Read the model definition and answer for the solid it produces. Units are mm, in the model's axes. Round coordinates to 2 decimals unless told otherwise and drop trailing zeros. Write each loop counter-clockwise with the first axis right and the second up, starting at its lowest first coordinate (ties: lowest second). Pieces come first, ordered by that corner, then holes.
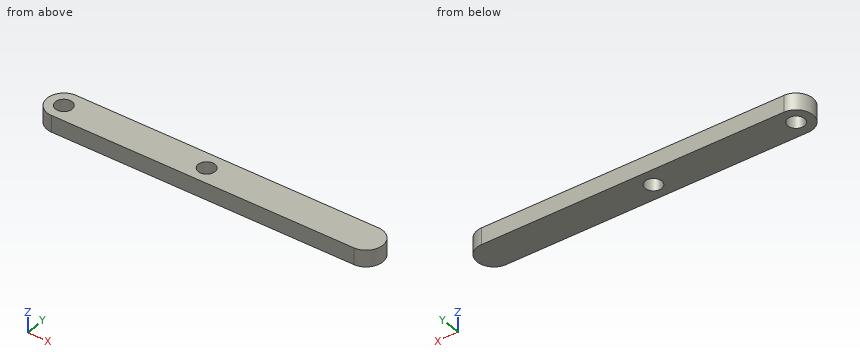
Autodesk Inventor part; units mm, degrees
ref_plane "YZ Plane" through (0, 0, 0) normal (1, 0, 0) x (0, 1, 0)
ref_plane "XZ Plane" through (0, 0, 0) normal (0, 1, 0) x (-1, 0, 0)
ref_plane "XY Plane" through (0, 0, 0) normal (0, 0, 1) x (1, 0, 0)
sketch "Skizze1" plane through (0, 0, 0) normal (0, 0, 1) x (1, 0, 0)
  line L0 (-25, 0) -> (115, 0)
  line L1 (0, -7) -> (0, 7)
  line L2 (0, 0) -> (90, 0) construction
  line L3 (0, -5) -> (90, -5)
  line L4 (90, 5) -> (0, 5)
  arc A0 (0, 5) -> (0, -5) centre (0, 0) ccw
  arc A1 (90, -5) -> (90, 5) centre (90, 0) ccw
  point P0 (45, 0)
  dimension "d0" = 90
  dimension "d1" = 10
extrude "Extrusion1" add sketch "Skizze1" along normal blind 5
sketch "Skizze2" plane through (0, 0, 5) normal (0, 0, 1) x (1, 0, 0)
  point P0 (0, 0)
  point P1 (0, 0)
hole "Bohrung1" at (0, 0, 5) direction (0, 0, -1) diameter 5 end through all
sketch "Skizze3" plane through (0, 0, 5) normal (0, 0, 1) x (1, 0, 0)
  point P0 (0, 0)
  point P1 (42.5, 0)
  dimension "d11" = 42.5
hole "Bohrung2" at (42.5, 0, 5) direction (0, 0, -1) diameter 5 end through all
properties part number "Hebel"
Q1. Straight lines are drawn through the part: probe 1 along X at (y, z) = (0, 3.25); probe 2 along X at (y, z) = (2.25, 3.45); probe 3 along Y at (x, z) = (0, 3.7). For each, find the intervals that lie inside material, in ascending order.
Verdict:
probe 1: x = -5 to -2.5, 2.5 to 40, 45 to 95
probe 2: x = -4.47 to -1.09, 1.09 to 41.41, 43.59 to 94.47
probe 3: y = -5 to -2.5, 2.5 to 5
Q2. Section C-C (x = 42.5) is taken. Determine the outline of the cut face in (y, z), then the cut area to 3 significant figures.
Verdict:
outline: (-5, 0) - (-2.5, 0) - (-2.5, 5) - (-5, 5) - close; (2.5, 0) - (5, 0) - (5, 5) - (2.5, 5) - close
area: 25.0 mm2
Q3. Section A-A (y = 0) is taken. Determine the outline of the cut face in (x, z), then the cut area to 3 significant figures.
Verdict:
outline: (-5, 0) - (-2.5, 0) - (-2.5, 5) - (-5, 5) - close; (2.5, 0) - (40, 0) - (40, 5) - (2.5, 5) - close; (45, 0) - (95, 0) - (95, 5) - (45, 5) - close
area: 450 mm2
Q4. Section B-B (z = 2.85) is taken. Determine the outline of the cut face in (x, y), then the cut area to 3 significant figures.
Verdict:
outline: (0, -5) - (90, -5) arc R5 ccw to (90, 5) - (0, 5) arc R5 ccw to start; hole circle Ø5 at (0, 0); hole circle Ø5 at (42.5, 0)
area: 939 mm2
Q5. Section D-D (y = -4) is taken. Determine the outline of the cut face in (x, z).
Verdict:
outline: (-3, 0) - (93, 0) - (93, 5) - (-3, 5) - close
